Build history of the part. All positions in model axes, mm. A direction names the side the tool comes from. Coordinates: 2 decimals unless noted, no trailing zeros. Loops run counter-clockwise (first coordinate to the right, second up) from the corner with the lowest first, then second, coordinate; pieces in that order, holes last. Notation, with made-up numbers: (26.25, -1.5) - (35.25, -1.5) arc R20 ccw to (35.25, 6.5) - close; hole circle Ø4 at (-15.75, 12.5). An arc over 180 degrees is marked (long way). One line per item, written item: value.
```python
from build123d import *

# Parameters (mm, degrees)
SKETCH3_R           = 7.5
BOSS_EXTRUDE1_DEPTH = 27.5
CHAMFER1_SIZE       = 0.75
FILLET2_R           = 0.5625
SKETCH4_W           = 1.2
SKETCH4_H           = 0.35


with BuildPart() as part:
    # Sketch3 → Boss-Extrude1 (new, symmetric)
    with BuildSketch(Plane.XY):
        Circle(SKETCH3_R)
    extrude(amount=BOSS_EXTRUDE1_DEPTH, both=True)

    # Chamfer1
    chamfer1_edges = [part.edges().sort_by_distance(p)[0] for p in [
        (-7.5, 0, -27.5),
        (-7.5, 0, 27.5),
    ]]
    chamfer(chamfer1_edges, length=CHAMFER1_SIZE)

    # Fillet2
    fillet2_edges = [part.edges().sort_by_distance(p)[0] for p in [
        (-7.5, 0, -26.75),
        (-7.5, 0, 26.75),
    ]]
    fillet(fillet2_edges, radius=FILLET2_R)

    # Sketch4 → Cut-Revolve1 (revolve, cut)
    with BuildSketch(Plane(origin=(0, 0, 0), x_dir=(0, 0, -1), z_dir=(1, 0, 0))):
        with Locations((25.1, 7.325)):
            Rectangle(SKETCH4_W, SKETCH4_H)
    cut_revolve1 = revolve(axis=Axis((0, 0, -27.5), (0, 0, 1)), mode=Mode.SUBTRACT)

    # Mirror1: Cut-Revolve1 across plane
    add(cut_revolve1.mirror(Plane.XY), mode=Mode.SUBTRACT)


solid = part.part
```
Item 1: Tool access for faces 1 (the face through (7.154, 2.253, 0.343)), 2 (the face through (-7.09, -0.93, 25.11)): list every direction of +Z, -Z, +X, -X, +Y, -Y with a clear straight run to the whole face (end or side of a thin tool).
Check result:
face 1: +Z, -Z
face 2: none
Item 2: Probe probe 1 along X at (y, z) = (-1.5, -18.5); probe 2 along X at (y, z) = (3.25, -15); probe 3 along Y at (x, z) = (2.25, -13). List the from-to ranges inside material, lowest first. Write a range as from..to.
Check result:
probe 1: x = -7.35..7.35
probe 2: x = -6.76..6.76
probe 3: y = -7.15..7.15
Item 3: Cut at A-A, the plane z = -2. Write the cut outline in (x, y), then the cut area to 3 significant figures.
Check result:
outline: circle Ø15 at (0, 0)
area: 177 mm^2
Item 4: Drop a flat-ended pin along its axis: P1, Ø2, axis at x = 4.5, z = -1.5, coming from the -Y side. Give the stop position or say it passes through.
Check result:
P1: stops at y = -6.63
